Geometry: final body of the model. Coordinates: model frame, mm. Face numbers are marked on the shaded views. Give positions to 0.01 mm unless a question says otherwise; leave off trailing zeros. Write each loop counter-clockwise with the first axis right and the second up, starting at its lowest first coordinate (ties: lowest second). Pieces come first, ordered by that corner, then holes. Notation, with made-up numbers: (42, 24) - (74, 24) arc R10 ccw to (74, 37) - close; hole circle Ø5 at (-28.75, 26). An arc over 180 degrees is marked (long way). Return JSON: item names as keys, results as strings.
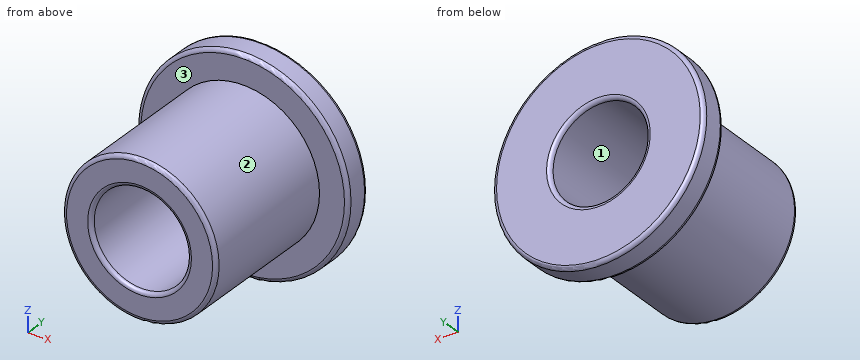
from build123d import *

# Parameters (mm, degrees)
F0_R     = 5.5
F1_DEPTH = 1.4
F2_R     = 4
F3_DEPTH = 7.6
F4_R     = 2.5
F5_DEPTH = 10
F6_R     = 0.2


with BuildPart() as f1:
    # F0 (on Front) → F1 (new body)
    with BuildSketch(Plane.XZ):
        Circle(F0_R)
    extrude(amount=F1_DEPTH)

    # F2 (on face) → F3 (join)
    with BuildSketch(Plane.XZ.offset(1.4)):
        Circle(F2_R)
    extrude(amount=F3_DEPTH)

    # F4 (on face) → F5 (cut)
    with BuildSketch(Plane.XZ.offset(9)):
        Circle(F4_R)
    extrude(amount=-F5_DEPTH, mode=Mode.SUBTRACT)

    # F6
    f6_edges = [f1.edges().sort_by_distance(p)[0] for p in [
        (-2.5, -9, 0),
        (-4, -9, 0),
        (-5.5, -1.4, 0),
        (-5.5, 0, 0),
        (-2.5, 0, 0),
    ]]
    fillet(f6_edges, radius=F6_R)


solid = f1.part
Q1. Mould query, pull axis X, two halves, no side actions, for the marked faces 1, 2 and 3. Classes: pulls with the +X half, pulls with the -X half, needs draft (parallel to the pull), parting line crosses it, or undercut.
Answer key:
{"face 1": "undercut", "face 2": "parting line crosses it", "face 3": "needs draft"}
Q2. Section query B-B, the plane x = 0. Return the cut outline in (y, z), plus the area to 3 significant figures.
Answer key:
{"outline": "(-9, -3.8) arc R0.2 ccw to (-8.8, -4) - (-1.4, -4) - (-1.4, -5.3) arc R0.2 ccw to (-1.2, -5.5) - (-0.2, -5.5) arc R0.2 ccw to (0, -5.3) - (0, -2.7) arc R0.2 ccw to (-0.2, -2.5) - (-8.8, -2.5) arc R0.2 ccw to (-9, -2.7) - close; (-9, 2.7) arc R0.2 ccw to (-8.8, 2.5) - (-0.2, 2.5) arc R0.2 ccw to (0, 2.7) - (0, 5.3) arc R0.2 ccw to (-0.2, 5.5) - (-1.2, 5.5) arc R0.2 ccw to (-1.4, 5.3) - (-1.4, 4) - (-8.8, 4) arc R0.2 ccw to (-9, 3.8) - close", "area": "31.1 mm^2"}
Q3. Section query C-C, the plane y = -6. Return the cut outline in (x, z).
Answer key:
{"outline": "circle Ø8 at (0, 0); hole circle Ø5 at (0, 0)"}
Q4. Section query A-A, the plane z = 0. Return the cut outline in (x, y), plus the area to 3 significant figures.
Answer key:
{"outline": "(-5.5, -1.2) arc R0.2 ccw to (-5.3, -1.4) - (-4, -1.4) - (-4, -8.8) arc R0.2 ccw to (-3.8, -9) - (-2.7, -9) arc R0.2 ccw to (-2.5, -8.8) - (-2.5, -0.2) arc R0.2 ccw to (-2.7, 0) - (-5.3, 0) arc R0.2 ccw to (-5.5, -0.2) - close; (2.5, -8.8) arc R0.2 ccw to (2.7, -9) - (3.8, -9) arc R0.2 ccw to (4, -8.8) - (4, -1.4) - (5.3, -1.4) arc R0.2 ccw to (5.5, -1.2) - (5.5, -0.2) arc R0.2 ccw to (5.3, 0) - (2.7, 0) arc R0.2 ccw to (2.5, -0.2) - close", "area": "31.1 mm^2"}
Q5. Material intervals for probe 1 along Z at (x, y) = (0, -3.75); probe 2 along Y at (x, z) = (-4.75, -1); probe 3 along Z at (x, y) = (1, -1.5), sorted ascending. Write a range as [from, to].
Answer key:
{"probe 1": "z = [-4, -2.5], [2.5, 4]", "probe 2": "y = [-1.4, 0]", "probe 3": "z = [-3.87, -2.29], [2.29, 3.87]"}
Q6. Pin query (flat end, axial travel): P1, Ø1.5, axis at x = 1.5, y = -3.5, coming from the +Z side; P2, Ø1.5, axis at x = 3.5, y = -7, coming from the +Z side; P3, Ø2, axis at x = 1, z = -1, coming from the +Y side; P4, Ø1, axis at x = 3.5, y = -4, coming from the -Z side. Return the tip coordinate at first contact, or that it passes through.
Answer key:
{"P1": "stops at z = 3.93", "P2": "stops at z = 2.9", "P3": "passes through", "P4": "stops at z = -2.65"}
